from build123d import *

# Parameters (mm, degrees)
BOSS_EXTRUDE1_DEPTH = 60
BOSS_EXTRUDE2_DEPTH = 10


with BuildPart() as part:
    # Sketch1 → Boss-Extrude1 (new body)
    with BuildSketch(Plane(origin=(0, 0, 0), x_dir=(1, 0, 0), z_dir=(0, 1, 0))):
        Polygon((-30, -12.426406871), (-12.426406871, -30), (-1.715728753, -30), (30, 1.715728753), (30, 12.426406871), (12.426406871, 30), (1.715728753, 30), (-30, -1.715728753), align=None)
    extrude(amount=BOSS_EXTRUDE1_DEPTH)

    # Sketch1_3 → Boss-Extrude2 (add)
    with BuildSketch(Plane(origin=(0, 0, 0), x_dir=(1, 0, 0), z_dir=(0, 1, 0))):
        Polygon((-30, -12.426406871), (-30, -30), (-12.426406871, -30), align=None)
        Polygon((30, 1.715728753), (-1.715728753, -30), (30, -30), align=None)
        Polygon((12.426406871, 30), (30, 12.426406871), (30, 30), align=None)
        Polygon((-30, 30), (-30, -1.715728753), (1.715728753, 30), align=None)
    extrude(amount=BOSS_EXTRUDE2_DEPTH)


solid = part.part
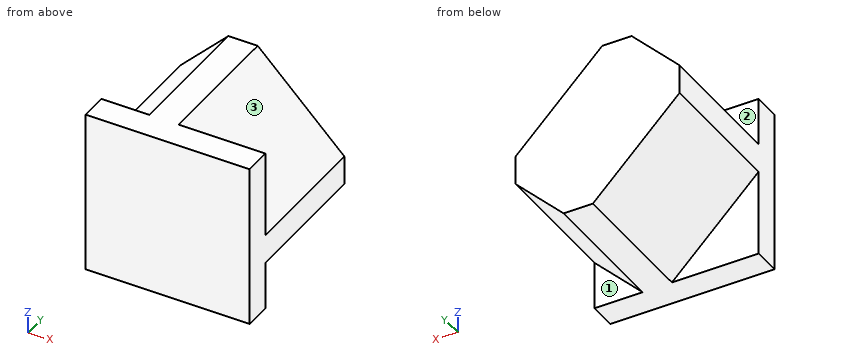
Design review of the part built by this model. Coordinates are the model's own, in mm. Face numbers are marked on the shaded views. A direction names the side the tool comes from. Give positions to 0.01 mm unless a question says otherwise; leave off trailing zeros. Write each loop counter-clockwise with the first axis right and the second up, starting at its lowest first coordinate (ties: lowest second). Pieces come first, ordered by that corner, then holes. Notation, with made-up numbers: M 47.25,2.25 L 98.25,2.25 A18 ccw 98.25,22.25 Z; hole C 31.5,21.5 d6. An arc over 180 degrees is marked long. Answer as a JSON object with one key per item and string values. Group by question number.
1) Clearance check with flat-ended pins moving along their axes: pin 1 Ø8 at (y, z) = (36, -19) entering from -X; pin 2 Ø5.5 at (x, z) = (22, -25) entering from +Y; pin 3 Ø4 at (x, y) = (7.5, 15.5) entering from +Z. State where each tip first meets the part, or that it passes through.
2) We need section A-A (y = 54). Give the boundary of the cut face in (x, z), and give its area (3 significant figures).
3) We need section B-B (x = -16.5). Give the boundary of the cut face in (y, z), and give its area (3 significant figures).
4) Tool access review of the marked faces 1, 2 and 3: name each direction out of +Z, -Z, +X, -X, +Y, -Y from which nothing blocks a thin tool from reaching the whole face with its end or side.
5) We need section C-C (z = 7). Give the boundary of the cut face in (x, y).
6) For line 1 along Y through (x, z) = (-26, -26); line 2 along Z through (x, y) = (27, 39); line 3 along Z through (x, y) = (21.5, 34.5), list the stretches that pass through material, from the lowest coordinate up.
7) We need section D-D (z = -8). Give the boundary of the cut face in (x, y).
Answer key:
{
 "1": {"pin 1": "stops at x = -13.28", "pin 2": "stops at y = 10", "pin 3": "stops at z = 22.78"},
 "2": {"outline": "M -30,1.72 L 1.72,-30 L 12.43,-30 L 30,-12.43 L 30,-1.72 L -1.72,30 L -12.43,30 L -30,12.43 Z", "area": "2,290 mm²"},
 "3": {"outline": "M 0,-30 L 10,-30 L 10,-11.78 L 60,-11.78 L 60,25.93 L 10,25.93 L 10,30 L 0,30 Z", "area": "2,490 mm²"},
 "4": {"face 1": "-Z, +X, +Y", "face 2": "+Z, -X, +Y", "face 3": "+Z, +X, +Y"},
 "5": {"outline": "M -30,0 L 30,0 L 30,10 L 21.28,10 L 21.28,60 L -30,60 Z"},
 "6": {"line 1": "y = 0 to 10", "line 2": "z = -15.43 to 1.28", "line 3": "z = -20.93 to 6.78"},
 "7": {"outline": "M -30,0 L 30,0 L 30,60 L -20.28,60 L -20.28,10 L -30,10 Z"}
}
